Print and shaded views of the part. All mm, measured from the part's lowest x, y and z. Round coordinates to 2 decimals unless told otherwise and drop trailing zeros. Loops run counter-clockwise (first coordinate to the right, second up) from the corner with the lowest first, then second, coordinate; pieces in that order, holes last. Notation, with made-up numbers: (-7.5, -9.75) - (5.5, -9.75) arc R20 ccw to (5.5, 18.25) - close; hole circle Ø6 at (-32.75, 22.25). An arc over 180 degrees is marked (long way). Answer as a JSON object with one key per item and string values.
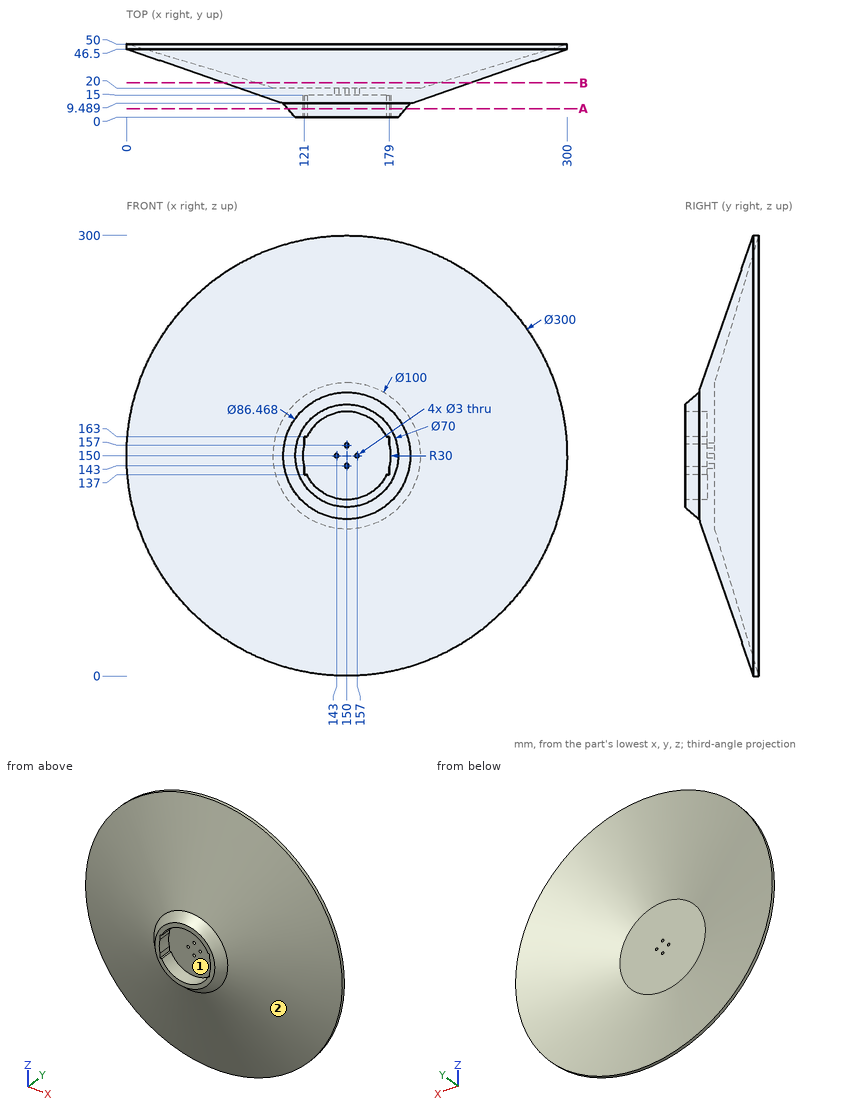
1) Slice it at A-A on y = 6. List the corners of the cut face in (x, z), then the cut area to 3 significant figures.
Values follow:
{"outline": "circle Ø80.41 at (150, 150); hole (121, 137) - (122.96, 137) arc R30 ccw to (177.04, 137) - (179, 137) - (179, 142.32) arc R30 ccw to (179, 157.68) - (179, 163) - (177.04, 163) arc R30 ccw to (122.96, 163) - (121, 163) - (121, 157.68) arc R30 ccw to (121, 142.32) - close", "area": "2,230 mm²"}
2) Two-plate mould, pull along Z, no slides. Class the marked faces 1 and 2: pulls with the +Z half, pulls with the -Z half, needs draft (parallel to the pull), parting line crosses it, or undercut.
Values follow:
{"face 1": "undercut", "face 2": "parting line crosses it"}
3) Drop flat-ended pins along their axis: P1, Ø3.5, axis at x = 150, z = 143, coming from the -Y side; P2, Ø5, axis at y = 5.5, z = 114.5, coming from the -X side (1 decimal); P3, Ø5, axis at x = 85.5, z = 252, coming from the -Y side. Give the stop position or say it passes through.
Values follow:
{"P1": "y = 15", "P2": "x = 126.2", "P3": "y = 35.47"}
4) Slice it at B-B on y = 23.5. List the corners of the cut face in (x, z), then the cut area to 3 significant figures.
Values follow:
{"outline": "circle Ø167.3 at (150, 150); hole circle Ø123.33 at (150, 150)", "area": "10,000 mm²"}
5) Probe probe 1 along Y at (x, z) = (150.5, 150); probe 2 along Y at (x, z) = (286, 183.5) (1 decimal). List the from-to ranges inside material, lowest first.
Values follow:
{"probe 1": "15 to 20", "probe 2": "43.1 to 47"}
